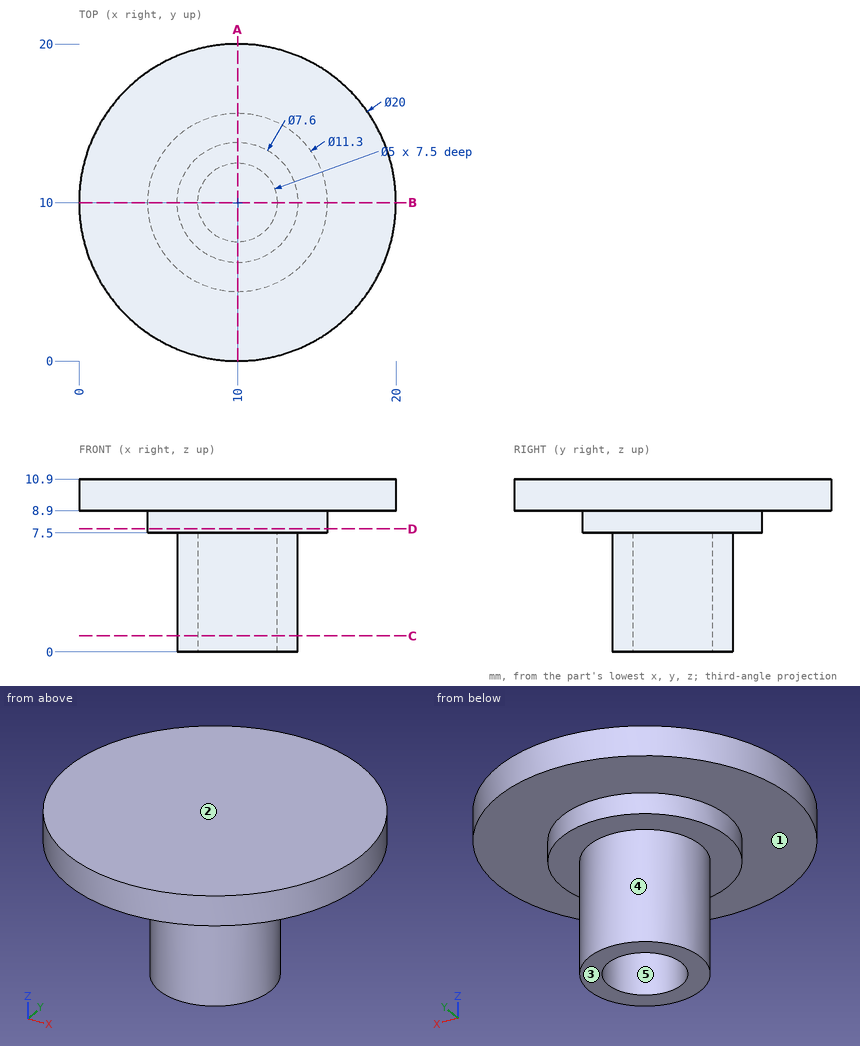
Part print with two shaded views. Sizes in mm from the minimum x, y, z corner. A direction names the side the tool comes from. Coordinates: 2 decimals unless noted, no trailing zeros. Write each loop counter-clockwise with the first axis right and the second up, starting at its lowest first coordinate (ties: lowest second). Pieces come first, ordered by that corner, then holes. Notation, with made-up numbers: (-0.75, 7) - (58.25, 7) arc R29 cw to (58.25, 34) - close; hole circle Ø9 at (-35.5, 73.25). An arc over 180 degrees is marked (long way). One line per item, written item: value. Start each with the question number.
1. Slice it at C-C (z = 1). Write the cut outline in (x, y).
2. Mould opens along Y. For the marked faces 3, 4 and 5 say: released by +Y, released by -Y, zero draft, split by the parting line, or undercut.
3. Probe line 1 (X direction, y = 10, z = 0.5); line 2 (Z direction, x = 11, y = 15). List the from-to ranges inside material, lowest first. Write a range as from..to.
4. Tool access for the marked faces 1 and 2: list every direction of +Z, -Z, +X, -X, +Y, -Y with a clear straight run to the whole face (end or side of a thin tool).
5. Slice it at A-A (x = 10). Write the cut outline in (y, z).
6. Slice it at D-D (z = 7.75). Write the cut outline in (x, y).
7. Flat gauge pins, fed straight in: pin 1 (5 mm diameter, centred on y = 17.5, z = 9, fed in from +X); pin 2 (2 mm diameter, centred on x = 13.5, z = 2.5, fed in from -Y); pin 3 (3 mm diameter, centred on x = 12, y = 4, fed in from -Z). Where does each tip first touch, or does it go through?
Answers below:
1. outline: circle Ø7.6 at (10, 10); hole circle Ø5 at (10, 10)
2. face 3: zero draft
2. face 4: split by the parting line
2. face 5: undercut
3. line 1: x = 6.2..7.5, 12.5..13.8
3. line 2: z = 7.5..10.9
4. face 1: -Z
4. face 2: +Z, +X, -X, +Y, -Y
5. outline: (0, 8.9) - (4.35, 8.9) - (4.35, 7.5) - (6.2, 7.5) - (6.2, 0) - (7.5, 0) - (7.5, 7.5) - (12.5, 7.5) - (12.5, 0) - (13.8, 0) - (13.8, 7.5) - (15.65, 7.5) - (15.65, 8.9) - (20, 8.9) - (20, 10.9) - (0, 10.9) - close
6. outline: circle Ø11.3 at (10, 10)
7. pin 1: stops at x = 18.66
7. pin 2: stops at y = 7.14
7. pin 3: stops at z = 7.5
